The model under review builds one solid part; all positions refer to its coordinate system, in mm. A direction names the side the tool comes from. Coordinates: 2 decimals unless noted, no trailing zeros. Loops run counter-clockwise (first coordinate to the right, second up) from the corner with the lowest first, then second, coordinate; pieces in that order, holes last. Notation, with made-up numbers: M 16,14 L 35,14 A16 ccw 35,43 Z; hole C 69,43 d4. An arc over 180 degrees is marked long. Return JSON: item names as keys, results as strings.
```python
from build123d import *

# Parameters (mm, degrees)
BOSS_EXTRUDE2_START       = -53.9167663
BOSS_EXTRUDE2_DEPTH       = 53.9167663
BOSS_EXTRUDE2_START_2     = -5.234980118
BOSS_EXTRUDE2_2_DEPTH     = 20.234980118
BOSS_EXTRUDE2_START_3     = -5.798989873
BOSS_EXTRUDE2_3_DEPTH     = 2.136888219
BOSS_EXTRUDE2_4_OUTLINE_W = 4
BOSS_EXTRUDE2_4_OUTLINE_H = 13
BOSS_EXTRUDE2_4_DEPTH     = 15
BOSS_EXTRUDE3_DEPTH       = 13
BOSS_EXTRUDE4_DEPTH       = 50
CUT_EXTRUDE2_DEPTH        = 91.086151296
BOSS_EXTRUDE12_REACH      = 92.086
CUT_EXTRUDE6_REACH        = 92.086


with BuildPart() as part:
    # Boss-Extrude2: read off the stored shape, not the designer's step
    # Boss-Extrude2 outline → Boss-Extrude2 (new body)
    with BuildSketch(Plane(origin=(0, 0, 0), x_dir=(1, 0, 0), z_dir=(0, 1, 0)).offset(BOSS_EXTRUDE2_START)):
        Polygon((0, -15), (0, 0), (-14, 5.798989873), (-14, -15), (-9, -15), (-9, -2), (-5, -2), (-5, -15), align=None)
    extrude(amount=BOSS_EXTRUDE2_DEPTH)



with BuildPart() as body_2:
    # Boss-Extrude2 2 outline → Boss-Extrude2 2 (new body)
    with BuildSketch(Plane.XY.offset(BOSS_EXTRUDE2_START_2)):
        Polygon((-14, 0), (0, 0), (-14, 14), align=None)
    extrude(amount=BOSS_EXTRUDE2_2_DEPTH)


with BuildPart() as part_1:
    add(part.part)

    add(body_2.part)  # Boss-Extrude2 3 merges body 2
    # Boss-Extrude2 3 outline → Boss-Extrude2 3 (add)
    with BuildSketch(Plane.XY.offset(BOSS_EXTRUDE2_START_3)):
        Polygon((-14, 0), (-9, 0), (-9, 9), (-14, 14), align=None)
    extrude(amount=BOSS_EXTRUDE2_3_DEPTH)

    # Boss-Extrude2 4 outline → Boss-Extrude2 4 (cut)
    with BuildSketch(Plane(origin=(0, 0, 0), x_dir=(1, 0, 0), z_dir=(0, 1, 0))):
        Polygon((0, 5.234980118), (-9, 5.234980118), (-9, 5.798989873), (-14, 5.798989873), (0, 0), align=None)
        with Locations((-7, -8.5)):
            Rectangle(BOSS_EXTRUDE2_4_OUTLINE_W, BOSS_EXTRUDE2_4_OUTLINE_H)
    extrude(amount=BOSS_EXTRUDE2_4_DEPTH, mode=Mode.SUBTRACT)

    # Sketch4 → Boss-Extrude3 (add)
    with BuildSketch(Plane.XY.offset(2)):
        Polygon((-5, 5), (-5, 3), (-9, 3), (-9, 9), align=None)
    extrude(amount=BOSS_EXTRUDE3_DEPTH)

    # Sketch5 → Boss-Extrude4 (add)
    with BuildSketch(Plane.XY.offset(15)):
        Polygon((-9, -10), (-9, 3), (-5, 3), (-5, -10), (0, -10), (0, 0), (-14, 14), (-14, -10), align=None)
    extrude(amount=BOSS_EXTRUDE4_DEPTH)

    # Sketch11 → Cut-Extrude2 (cut, through all)
    with BuildSketch(Plane.XY.offset(65)):
        Polygon((-9.899494937, 9.899494937), (-14, 5.798989873), (-14, 14), align=None)
    extrude(amount=-CUT_EXTRUDE2_DEPTH, mode=Mode.SUBTRACT)

    # Boss-Extrude12: up to this plane
    boss_extrude12_end = Plane(origin=(0, -53.9167663, 0), z_dir=(0.38268343236508406, 0, -0.9238795325112893))
    # Sketch21 → Boss-Extrude12 (add, up to the surface)
    with BuildSketch(Plane.XY.offset(65), mode=Mode.PRIVATE) as boss_extrude12_sk1:
        Polygon((-9.899494937, 9.899494937), (-9.192388155, 10.606601718), (0.707106781, 0.707106781), (0, 0), align=None)
    boss_extrude12_tool1 = split(extrude(boss_extrude12_sk1.sketch, amount=-BOSS_EXTRUDE12_REACH, mode=Mode.PRIVATE), bisect_by=boss_extrude12_end, keep=Keep.BOTH, mode=Mode.PRIVATE)
    add(boss_extrude12_tool1.solids().sort_by_distance((-4.596194, 5.303301, 65))[0])

    # Cut-Extrude6: up to this plane
    cut_extrude6_end = Plane(origin=(0, -53.9167663, 0), z_dir=(0.38268343236508406, 0, -0.9238795325112893))
    # Sketch22 → Cut-Extrude6 (cut, up to the surface)
    with BuildSketch(Plane.XY.offset(65), mode=Mode.PRIVATE) as cut_extrude6_sk1:
        Polygon((-3.429467889, 2.015254326), (-2.015254326, 3.429467889), (-3.641599923, 5.055813485), (-5.055813485, 3.641599923), align=None)
    cut_extrude6_tool1 = split(extrude(cut_extrude6_sk1.sketch, amount=-CUT_EXTRUDE6_REACH, mode=Mode.PRIVATE), bisect_by=cut_extrude6_end, keep=Keep.BOTH, mode=Mode.PRIVATE)
    add(cut_extrude6_tool1.solids().sort_by_distance((-3.535534, 3.535534, 65))[0], mode=Mode.SUBTRACT)
    # Sketch22 → Cut-Extrude6 (cut, up to the surface)
    with BuildSketch(Plane.XY.offset(65), mode=Mode.PRIVATE) as cut_extrude6_sk2:
        Polygon((-6.257895014, 4.843681451), (-4.843681451, 6.257895014), (-6.470027048, 7.88424061), (-7.88424061, 6.470027048), align=None)
    cut_extrude6_tool2 = split(extrude(cut_extrude6_sk2.sketch, amount=-CUT_EXTRUDE6_REACH, mode=Mode.PRIVATE), bisect_by=cut_extrude6_end, keep=Keep.BOTH, mode=Mode.PRIVATE)
    add(cut_extrude6_tool2.solids().sort_by_distance((-6.363961, 6.363961, 65))[0], mode=Mode.SUBTRACT)


solid = part_1.part
```
1. Add section B-B on y = -8. Give the boundary of the cut face in (x, z), plus the area to 3 significant figures.
Check values:
{"outline": "M -14,-5.8 L 0,0 L 0,65 L -5,65 L -5,2 L -9,2 L -9,65 L -14,65 Z", "area": "699 mm²"}
2. To check wall thickness, follow line 1 (X direction, y = 0, z = 50); line 2 (Z direction, x = -2, y = -44); line 3 (Y direction, x = -3.75, z = 60). State the ranges of each line that lie inside material, in increasing order.
Check values:
{"line 1": "-14 to -9, -5 to 0", "line 2": "-0.83 to 15", "line 3": "-10 to 2.34, 4.95 to 5.16"}
3. Add section C-C on z = 56. Give the boundary of the cut face in (x, y).
Check values:
{"outline": "M -14,-10 L -9,-10 L -9,3 L -5,3 L -5,-10 L 0,-10 L 0,0 L 0.71,0.71 L -2.02,3.43 L -3.43,2.02 L -5.06,3.64 L -3.64,5.06 L -4.84,6.26 L -6.26,4.84 L -7.88,6.47 L -6.47,7.88 L -9.19,10.61 L -14,5.8 Z"}
4. Insertion check: pin 1 Ø5.5 at (x, z) = (-2, 46.5) entering from -Y; pin 2 Ø5.5 at (x, y) = (-12.5, -26.5) entering from +Z; pin 3 Ø6 at (x, z) = (-5.5, 47) entering from +Y. Each pin has a flat end and moves straight along its axis. Give the tip position at first contact, or say it passes through.
Check values:
{"pin 1": "y = -10", "pin 2": "z = 15", "pin 3": "y = 9.91"}
5. Machinability: for faces 4 (the face through (-5, -6, 19)), 5 (the face through (-11, -32, 15)), 6 (the face through (-0.673, 2.087, 32.543)), 7 (the face through (-14, -17, 13)), 8 (the face through (-7.082, 5.668, 31.345)), which of the approach directions +Z, -Z, +X, -X, +Y, -Y give a long, thin tool a straight path to every point of the face, cutting with its end or side? Answer none if there is none.
Check values:
{"face 4": "+Z, -Y", "face 5": "+Z, +X, -X, -Y", "face 6": "+Z, -Z, +X, +Y", "face 7": "+Z, -Z, -X, +Y, -Y", "face 8": "+Z, -Z"}
6. Add section A-A on z = 11.5. Give the boundary of the cut face in (x, y).
Check values:
{"outline": "M -14,-53.92 L -9,-53.92 L -9,3 L -5,3 L -5,-53.92 L 0,-53.92 L 0,0 L 0.71,0.71 L -2.02,3.43 L -3.43,2.02 L -5.06,3.64 L -3.64,5.06 L -4.84,6.26 L -6.26,4.84 L -7.88,6.47 L -6.47,7.88 L -9.19,10.61 L -14,5.8 Z"}
7. Add section D-D on x = -12.25. Give the boundary of the cut face in (y, z).
Check values:
{"outline": "M -53.92,-5.07 L 7.55,-5.07 L 7.55,65 L -10,65 L -10,15 L -53.92,15 Z"}
8. The part is to be moulded in two halves that separate along X. For faces 1 (the face through (0, -9, 18)), 2 (the face through (-10, -2, 65)), 3 (the face through (-7, -26, 2)), say which applies: released by +X, released by -X, zero draft, split by the parting line, or undercut.
Check values:
{"face 1": "released by +X", "face 2": "zero draft", "face 3": "undercut"}
